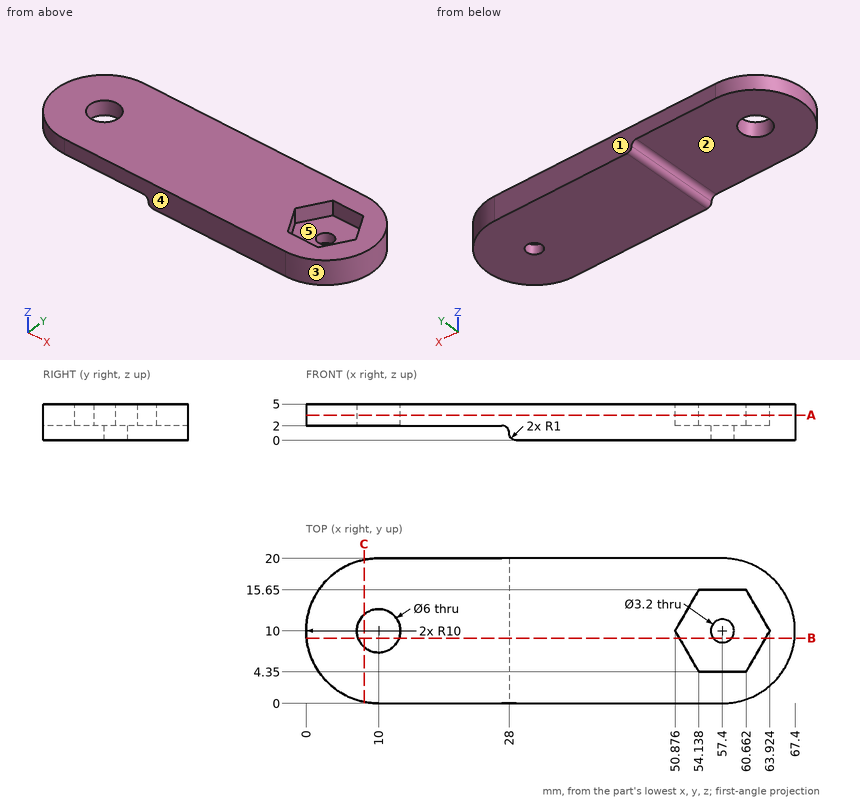
Drawing for the job (mm, zero at the part's lowest x, y, z). A direction names the side the tool comes from. Round coordinates to 2 decimals unless told otherwise and drop trailing zeros. Write each loop counter-clockwise with the first axis right and the second up, starting at its lowest first coordinate (ties: lowest second). Pieces come first, ordered by that corner, then holes. Notation, with made-up numbers: M 17,80.25 L 64,80.25 A14 ccw 64,84.25 Z; hole C 15.25,26.5 d4. An arc over 180 degrees is marked long. Answer as a JSON object with one key per item and string values. Group by question number.
(1) Which spindle directions (+Z, -Z, +X, -X, +Y, -Y) get a long thin tool onto all of the face, cutting with end or side? Do the marked faces 1 and 2. Say none if no direction does.
(2) Cut at A-A (z = 3.45). Give the cut face in (x, y).
(3) Cut at B-B (y = 9). Give the number of separate pieces and of enclosed holes in the cut face, and give its area (3 significant figures).
(4) Cut at C-C (x = 8). Give the cut face in (y, z).
(5) Flat gauge pins, fed straight in: pin 1 (5 mm diameter, centred on x = 57.4, y = 10, fed in from +Z); pin 2 (3 mm diameter, centred on y = 12, z = 4, fed in from -X); pin 3 (1 mm diameter, centred on y = 7.5, z = 1, fed in from -X). Where does each tip first touch, or does it go through?
(6) Drill centre lines: L1, parallel to X at y = 10, z = 2.7; L2, parallel to Y at x = 57.4, z = 1.5; L3, parallel to Y at x = 61.5, z = 4.5. Where is each one in solid material? Low to high.
(7) Mould opens along Y. For the marked faces 3, 4 and 5 say: pulls with the +Y half, pulls with the -Y half, needs draft (parallel to the pull), parting line crosses it, or undercut.
Responses:
{
 "1": {"face 1": "+Z, -Z, +X, -X, +Y", "face 2": "-Z, -X, +Y, -Y"},
 "2": {"outline": "M 10,0 L 57.4,0 A10 ccw 57.4,20 L 10,20 A10 ccw Z; hole C 10,10 d6; hole M 50.88,10 L 54.14,4.35 L 60.66,4.35 L 63.92,10 L 60.66,15.65 L 54.14,15.65 Z"},
 "3": {"separate pieces": "3", "enclosed holes": "0", "area": "223 mm2"},
 "4": {"outline": "M 0.2,2 L 7.76,2 L 7.76,5 L 0.2,5 Z; M 12.24,2 L 19.8,2 L 19.8,5 L 12.24,5 Z"},
 "5": {"pin 1": "stops at z = 2", "pin 2": "stops at x = 0.01", "pin 3": "stops at x = 27.87"},
 "6": {"L1": "x = 0 to 7, 13 to 50.88, 63.92 to 67.4", "L2": "y = 0 to 8.4, 11.6 to 20", "L3": "y = 0.88 to 5.8, 14.2 to 19.12"},
 "7": {"face 3": "parting line crosses it", "face 4": "pulls with the -Y half", "face 5": "undercut"}
}
